Source: CAD feature listing. Evaluate the final solid. Frame: model axes, mm. Round coordinates to 2 decimals unless told otherwise and drop trailing zeros. Write each loop counter-clockwise with the first axis right and the second up, starting at its lowest first coordinate (ties: lowest second). Pieces come first, ordered by that corner, then holes. Notation, with made-up numbers: M 62.25,7.25 L 116.25,7.25 A19 cw 116.25,22.25 Z; hole C -29.5,52.25 d7. An arc over 180 degrees is marked long. Use a Markdown table: item, result.
```python
from build123d import *

# Parameters (mm, degrees)
BOSS_EXTRUDE1_DEPTH = 308.00000001
CUT_EXTRUDE1_REACH  = 310.829
SKETCH2_R           = 0.889


with BuildPart() as part:
    # Sketch1 → Boss-Extrude1 (new body)
    with BuildSketch(Plane.XY):
        with BuildLine():
            Line((-19.689777646, 0), (19.689777646, 0))
            ThreePointArc((19.689777646, 0), (0, 11.1125), (-19.689777646, 0))
        make_face()
    extrude(amount=BOSS_EXTRUDE1_DEPTH)

    # Sketch2 → Cut-Extrude1 (cut, up to next)
    with BuildSketch(Plane.XY.offset(308.00000001), mode=Mode.PRIVATE) as cut_extrude1_sk1:
        with Locations((-11.269696042, 2.799461)):
            Circle(SKETCH2_R)
    cut_extrude1_tool1 = extrude(cut_extrude1_sk1.sketch, amount=-CUT_EXTRUDE1_REACH, mode=Mode.PRIVATE) & part.part
    # Sketch2 → Cut-Extrude1 (cut, up to next)
    with BuildSketch(Plane.XY.offset(308.00000001), mode=Mode.PRIVATE) as cut_extrude1_sk2:
        with Locations((-7.084427042, 5.2158138)):
            Circle(SKETCH2_R)
    cut_extrude1_tool2 = extrude(cut_extrude1_sk2.sketch, amount=-CUT_EXTRUDE1_REACH, mode=Mode.PRIVATE) & part.part
    # Sketch2 → Cut-Extrude1 (cut, up to next)
    with BuildSketch(Plane.XY.offset(308.00000001), mode=Mode.PRIVATE) as cut_extrude1_sk3:
        with Locations((-2.416366133, 6.4666114)):
            Circle(SKETCH2_R)
    cut_extrude1_tool3 = extrude(cut_extrude1_sk3.sketch, amount=-CUT_EXTRUDE1_REACH, mode=Mode.PRIVATE) & part.part
    # Sketch2 → Cut-Extrude1 (cut, up to next)
    with BuildSketch(Plane.XY.offset(308.00000001), mode=Mode.PRIVATE) as cut_extrude1_sk4:
        with Locations((2.416366133, 6.4666114)):
            Circle(SKETCH2_R)
    cut_extrude1_tool4 = extrude(cut_extrude1_sk4.sketch, amount=-CUT_EXTRUDE1_REACH, mode=Mode.PRIVATE) & part.part
    # Sketch2 → Cut-Extrude1 (cut, up to next)
    with BuildSketch(Plane.XY.offset(308.00000001), mode=Mode.PRIVATE) as cut_extrude1_sk5:
        with Locations((7.084427042, 5.2158138)):
            Circle(SKETCH2_R)
    cut_extrude1_tool5 = extrude(cut_extrude1_sk5.sketch, amount=-CUT_EXTRUDE1_REACH, mode=Mode.PRIVATE) & part.part
    # Sketch2 → Cut-Extrude1 (cut, up to next)
    with BuildSketch(Plane.XY.offset(308.00000001), mode=Mode.PRIVATE) as cut_extrude1_sk6:
        with Locations((11.269695955, 2.799461)):
            Circle(SKETCH2_R)
    cut_extrude1_tool6 = extrude(cut_extrude1_sk6.sketch, amount=-CUT_EXTRUDE1_REACH, mode=Mode.PRIVATE) & part.part
    add(cut_extrude1_tool1.solids().sort_by_distance((-11.269696, 2.799461, 308))[0], mode=Mode.SUBTRACT)
    add(cut_extrude1_tool2.solids().sort_by_distance((-7.084427, 5.215814, 308))[0], mode=Mode.SUBTRACT)
    add(cut_extrude1_tool3.solids().sort_by_distance((-2.416366, 6.466611, 308))[0], mode=Mode.SUBTRACT)
    add(cut_extrude1_tool4.solids().sort_by_distance((2.416366, 6.466611, 308))[0], mode=Mode.SUBTRACT)
    add(cut_extrude1_tool5.solids().sort_by_distance((7.084427, 5.215814, 308))[0], mode=Mode.SUBTRACT)
    add(cut_extrude1_tool6.solids().sort_by_distance((11.269696, 2.799461, 308))[0], mode=Mode.SUBTRACT)


solid = part.part
```
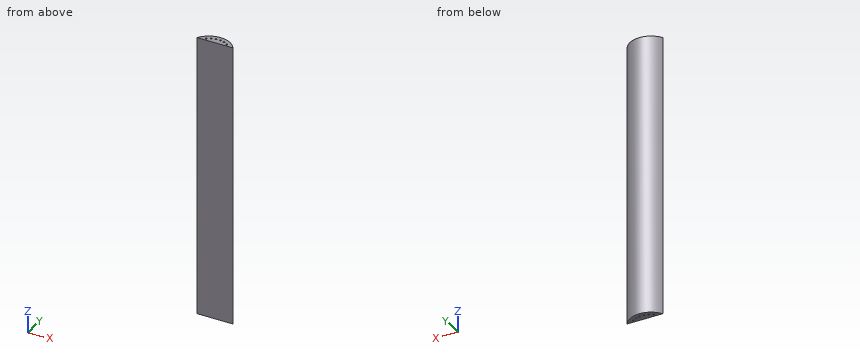
Q1. Line query: L1, parallel to X at y = 6.5, z = 226; L2, parallel to X at y = 7, z = 77; L3, parallel to Y at x = 0.5, z = 66. Output: solid intervals per line, ascending.
Results are:
| item | result |
|---|---|
| L1 | -13.82 to -3.3, -1.53 to 1.53, 3.3 to 13.82 |
| L2 | -13.12 to -3.13, -1.71 to 1.71, 3.13 to 13.12 |
| L3 | 0 to 11.11 |
Q2. First-contact query: pin 1 Ø4 at (y, z) = (3.5, 270.5) entering from +X; pin 2 Ø5 at (y, z) = (7.5, 157) entering from +X. Flat tips, straight axial feed; report the tip coordinate or a pass-through.
Results are:
| item | result |
|---|---|
| pin 1 | x = 18.7 |
| pin 2 | x = 15.61 |
Q3. Section A-A on z = 178.5. Return loops of the section in (x, y).
Results are:
| item | result |
|---|---|
| outline | M -19.69,0 L 19.69,0 A23 ccw Z; hole C -11.27,2.8 d1.78; hole C -7.08,5.22 d1.78; hole C -2.42,6.47 d1.78; hole C 2.42,6.47 d1.78; hole C 7.08,5.22 d1.78; hole C 11.27,2.8 d1.78 |
Q4. Section C-C on x = 16. Return loops of the section in (y, z), plus the area to 3 significant figures.
Results are:
| item | result |
|---|---|
| outline | M 0,0 L 4.64,0 L 4.64,308 L 0,308 Z |
| area | 1,430 mm^2 |
Q5. Section B-B on y = 9.25. Return loops of the section in (x, z), plus the area to 3 significant figures.
Results are:
| item | result |
|---|---|
| outline | M -9.07,0 L 9.07,0 L 9.07,308 L -9.07,308 Z |
| area | 5,590 mm^2 |
